Design review of the part built by this model. Coordinates are the model's own, in mm. Coordinates: 2 decimals unless noted, no trailing zeros. Loops run counter-clockwise (first coordinate to the right, second up) from the corner with the lowest first, then second, coordinate; pieces in that order, holes last.
Q1. For P1, Ø0.5, axis at x = 9, z = 5.5, coming from the -Y side; P2, Ø0.8, axis at x = 5, z = 5.5, coming from the +Y side; P3, Ø1.5, axis at x = -26, z = 4.5, coming from the -Y side, all flat-tipped, find the tip position at first contact; note any pin that passes through.
Q2. Add section B-B on y = -49. Give the boundary of the cut face in (x, z), and give its area (3 significant figures).
Q3. Add section D-D on x = -8.5. Give the boundary of the cut face in (y, z).
Q4. Add section A-A on z = 2.6. Give the boundary of the cut face in (x, y).
Q5. Add section C-C on x = 41.5. Give the boundary of the cut face in (y, z), and give its area (3 significant figures).
Q6. Wall thickness on probe 1 along Z at (x, y) = (30, 28.5); probe 2 along Y at (x, z) = (3, 5.7); probe 3 along X at (y, z) = (-20, 4.7): over which ranges is each line inside the solid? List them lowest first.
```python
from build123d import *

# Parameters (mm, degrees)
F1_DEPTH = 5
F2_DEPTH = 6


# Not quite as in the source:
# - a feature names something its author has since deleted; it is built from what else it names


with BuildPart() as f1:
    # F0 (on Top) → F1 (new body)
    with BuildSketch(Plane.XY):
        Polygon((25, 78.4878924489), (0, 78.4878924489), (-25, 78.4878924489), (-13.1142183076, 25.3134854138), (-56.342728436, 39.404849359), (-56.342728436, -10.595150641), (-13.1142183076, 0), (-25, -121.5121075511), (0, -121.5121075511), (25, -121.5121075511), (13.1142183076, 0), (56.342728436, -10.595150641), (56.342728436, 39.404849359), (13.1142183076, 25.3134854138), align=None)
        Polygon((-18.0415231461, 71.7220325265), (0, 71.7220325265), (18.0415231461, 71.7220325265), (5.9721833782, 17.7264265097), (51.342728436, 32.5160378311), (51.342728436, -4.2216783711), (5.9721833782, 5.9197491293), (17.9479308986, -116.5121075511), (0, -116.5121075511), (-17.9479308986, -116.5121075511), (-5.9721833782, 5.9197491293), (-51.342728436, -4.2216783711), (-51.342728436, 32.5160378311), (-5.9721833782, 17.7264265097), align=None, mode=Mode.SUBTRACT)
        Polygon((18.0415231461, 71.7220325265), (0, 71.7220325265), (-18.0415231461, 71.7220325265), (-5.9721833782, 17.7264265097), (-51.342728436, 32.5160378311), (-51.342728436, -4.2216783711), (-5.9721833782, 5.9197491293), (-17.9479308986, -116.5121075511), (0, -116.5121075511), (17.9479308986, -116.5121075511), (5.9721833782, 5.9197491293), (51.342728436, -4.2216783711), (51.342728436, 32.5160378311), (5.9721833782, 17.7264265097), align=None)
    extrude(amount=F1_DEPTH)

    # F0 (on Top) → F2 (join)
    with BuildSketch(Plane.XY):
        Polygon((18.0415231461, 71.7220325265), (0, 71.7220325265), (-18.0415231461, 71.7220325265), (-5.9721833782, 17.7264265097), (-51.342728436, 32.5160378311), (-51.342728436, -4.2216783711), (-5.9721833782, 5.9197491293), (-17.9479308986, -116.5121075511), (0, -116.5121075511), (17.9479308986, -116.5121075511), (5.9721833782, 5.9197491293), (51.342728436, -4.2216783711), (51.342728436, 32.5160378311), (5.9721833782, 17.7264265097), align=None)
    extrude(amount=F2_DEPTH)


solid = f1.part
```
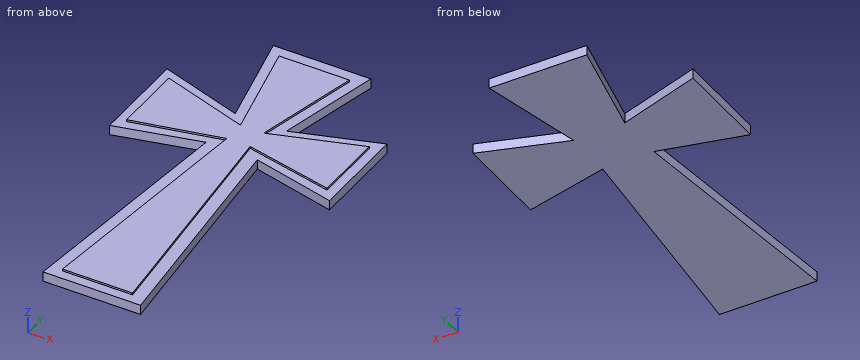
Entries:
1. P1: stops at y = -116.51
1. P2: stops at y = 71.72
1. P3: stops at y = -3.34
2. outline: (-17.91, 0) - (17.91, 0) - (17.91, 5) - (11.34, 5) - (11.34, 6) - (-11.34, 6) - (-11.34, 5) - (-17.91, 5) - close
2. area: 202 mm2
3. outline: (-121.51, 0) - (78.49, 0) - (78.49, 5) - (71.72, 5) - (71.72, 6) - (29.04, 6) - (29.04, 5) - (18.55, 5) - (18.55, 6) - (5.35, 6) - (5.35, 5) - (-19.92, 5) - (-19.92, 6) - (-116.51, 6) - (-116.51, 5) - (-121.51, 5) - close
4. outline: (-56.34, -10.6) - (-13.11, 0) - (-25, -121.51) - (25, -121.51) - (13.11, 0) - (56.34, -10.6) - (56.34, 39.4) - (13.11, 25.31) - (25, 78.49) - (-25, 78.49) - (-13.11, 25.31) - (-56.34, 39.4) - close
5. outline: (-6.96, 0) - (34.57, 0) - (34.57, 5) - (29.31, 5) - (29.31, 6) - (-2.02, 6) - (-2.02, 5) - (-6.96, 5) - close
5. area: 239 mm2
6. probe 1: z = 0 to 5
6. probe 2: y = -116.51 to 71.72
6. probe 3: x = -15.07 to 15.07
